Design review of the part built by this model. Coordinates are the model's own, in mm. A direction names the side the tool comes from. Coordinates: 2 decimals unless noted, no trailing zeros. Order: outer loops, then holes, each group sorted by start corner. A loop starts at its lowest first (then second) coordinate and runs counter-clockwise, first axis right, second up. Notation, with made-up numbers: M 89,69 L 135,69 A18 ccw 135,94 Z; hole C -25,7.5 d10. An arc over 180 degrees is marked long. Answer in a Markdown table with one row per item.
from build123d import *

# Parameters (mm, degrees)
SKETCH1_W            = 90.57
SKETCH1_H            = 65.6
BOSS_EXTRUDE1_DEPTH  = 1
SKETCH2_R            = 1.3
CUT_EXTRUDE1_DEPTH   = 112.835973193
SKETCH3_W            = 10.14
SKETCH3_H            = 10.14
SKETCH3_W_2          = 30.4
BOSS_EXTRUDE2_DEPTH  = 8
SKETCH4_W            = 14.4
SKETCH4_H            = 10.82
BOSS_EXTRUDE3_DEPTH  = 6
SKETCH5_W            = 9
SKETCH5_H            = 12
BOSS_EXTRUDE4_DEPTH  = 11
FILLET2_R            = 4.5
SKETCH7_W            = 9
SKETCH7_H            = 3
BOSS_EXTRUDE5_DEPTH  = 11
SKETCH8_R            = 4
BOSS_EXTRUDE6_DEPTH  = 9
SKETCH9_W            = 22.948138565
SKETCH9_H            = 3.071798075
SKETCH9_W_2          = 9.215394227
SKETCH9_H_2          = 3.975268097
SKETCH9_W_3          = 5.149779126
SKETCH9_H_3          = 20.147381496
SKETCH9_W_4          = 3.975268098
SKETCH9_H_4          = 8.94435322
SKETCH9_H_5          = 11.519242784
BOSS_EXTRUDE7_DEPTH  = 5
SKETCH10_W           = 17.979053442
SKETCH10_H           = 12.196845301
BOSS_EXTRUDE8_DEPTH  = 1
SKETCH12_W           = 26.83305966
SKETCH12_H           = 5.142650184
BOSS_EXTRUDE9_DEPTH  = 2.5
SKETCH13_W           = 30.989021763
SKETCH13_H           = 4.427003109
BOSS_EXTRUDE10_DEPTH = 5


with BuildPart() as part:
    # Sketch1 → Boss-Extrude1 (new body)
    with BuildSketch(Plane(origin=(0, 0, 0), x_dir=(1, 0, 0), z_dir=(0, 1, 0))):
        with Locations((45.285, 32.8)):
            Rectangle(SKETCH1_W, SKETCH1_H)
    extrude(amount=BOSS_EXTRUDE1_DEPTH)

    # Sketch2 → Cut-Extrude1 (cut, through all)
    with BuildSketch(Plane(origin=(0, 1, 0), x_dir=(1, 0, 0), z_dir=(0, 1, 0))):
        with Locations(Location((2.36, 2.31, 0), (0, 0, 270))):
            Circle(SKETCH2_R)
        with Locations(Location((3.099, 62.1, 0), (0, 0, 270))):
            Circle(SKETCH2_R)
        with Locations(Location((88.7, 61.87, 0), (0, 0, 270))):
            Circle(SKETCH2_R)
        with Locations(Location((79.55, 1.49, 0), (0, 0, 270))):
            Circle(SKETCH2_R)
    extrude(amount=-CUT_EXTRUDE1_DEPTH, mode=Mode.SUBTRACT)

    # Sketch3 → Boss-Extrude2 (add)
    with BuildSketch(Plane(origin=(0, 1, 0), x_dir=(1, 0, 0), z_dir=(0, 1, 0))):
        with Locations((10.91, 62.53)):
            Rectangle(SKETCH3_W, SKETCH3_H)
        with Locations((33.46, 62.53)):
            Rectangle(SKETCH3_W_2, SKETCH3_H)
    extrude(amount=BOSS_EXTRUDE2_DEPTH)

    # Sketch4 → Boss-Extrude3 (add)
    with BuildSketch(Plane(origin=(0, 1, 0), x_dir=(1, 0, 0), z_dir=(0, 1, 0))):
        with Locations((59.95, 60.19)):
            Rectangle(SKETCH4_W, SKETCH4_H)
    extrude(amount=BOSS_EXTRUDE3_DEPTH)

    # Sketch5 → Boss-Extrude4 (add)
    with BuildSketch(Plane(origin=(0, 1, 0), x_dir=(1, 0, 0), z_dir=(0, 1, 0))):
        with Locations((81.97, 59.6)):
            Rectangle(SKETCH5_W, SKETCH5_H)
    extrude(amount=BOSS_EXTRUDE4_DEPTH)

    # Fillet2
    fillet2_edges = [part.edges().sort_by_distance(p)[0] for p in [
        (86.47, 12, -59.6),
        (77.47, 12, -59.6),
    ]]
    fillet(fillet2_edges, radius=FILLET2_R - 0.0001)  # a hair under: the kernel refuses the full size

    # Sketch7 → Boss-Extrude5 (add)
    with BuildSketch(Plane(origin=(0, 1, 0), x_dir=(1, 0, 0), z_dir=(0, 1, 0))):
        with Locations((81.97, 67.1)):
            Rectangle(SKETCH7_W, SKETCH7_H)
    extrude(amount=BOSS_EXTRUDE5_DEPTH)

    # Sketch8 → Boss-Extrude6 (add)
    with BuildSketch(Plane(origin=(0, 0, -67.6), x_dir=(-1, 0, 0), z_dir=(0, 0, -1))):
        with Locations(Location((-10.91, 5, 0), (0, 0, 270))):
            Circle(SKETCH8_R)
    extrude(amount=BOSS_EXTRUDE6_DEPTH)

    # Sketch9 → Boss-Extrude7 (add)
    with BuildSketch(Plane(origin=(0, 1, 0), x_dir=(1, 0, 0), z_dir=(0, 1, 0))):
        with Locations((34.443359734, 53.839684383)):
            Rectangle(SKETCH9_W, SKETCH9_H)
        with Locations((11.404874166, 47.334700223)):
            Rectangle(SKETCH9_W_2, SKETCH9_H_2)
        with Locations((6.661656549, 22.263407105)):
            Rectangle(SKETCH9_W_3, SKETCH9_H_3)
        with Locations((83.953516952, 39.248643523)):
            Rectangle(SKETCH9_W_4, SKETCH9_H_4)
        with Locations((83.953516952, 28.023028497)):
            Rectangle(SKETCH9_W_4, SKETCH9_H_5)
    extrude(amount=BOSS_EXTRUDE7_DEPTH)

    # Sketch10 → Boss-Extrude8 (add)
    with BuildSketch(Plane(origin=(0, 1, 0), x_dir=(1, 0, 0), z_dir=(0, 1, 0))):
        with Locations((39.18657735, 33.647129386)):
            Rectangle(SKETCH10_W, SKETCH10_H)
    extrude(amount=BOSS_EXTRUDE8_DEPTH)

    # Sketch12 → Boss-Extrude9 (add)
    with BuildSketch(Plane(origin=(0, 1, 0), x_dir=(1, 0, 0), z_dir=(0, 1, 0))):
        with Locations((32.862287194, 2.571325092)):
            Rectangle(SKETCH12_W, SKETCH12_H)
    extrude(amount=BOSS_EXTRUDE9_DEPTH)

    # Sketch13 → Boss-Extrude10 (add)
    with BuildSketch(Plane(origin=(0, 1, 0), x_dir=(1, 0, 0), z_dir=(0, 1, 0))):
        with Locations((39.186577349, 19.462650037)):
            Rectangle(SKETCH13_W, SKETCH13_H)
    extrude(amount=BOSS_EXTRUDE10_DEPTH)


solid = part.part
(1) Add section C-C, the plane x = 59. Give the boundary of the cut face in (y, z).
Return value:
| item | result |
|---|---|
| outline | M 0,-65.6 L 7,-65.6 L 7,-54.78 L 1,-54.78 L 1,0 L 0,0 Z |
(2) For line 1 along X through (y, z) = (0.4, -62.1); line 2 along X through (y, z) = (0.7, -2.31); line 3 along Z through (x, y) = (79.55, 0.5), list the stretches that pass through material, from the lowest coordinate up. Write a range as from..to.
Return value:
| item | result |
|---|---|
| line 1 | x = 0..1.8, 4.4..87.42, 89.98..90.57 |
| line 2 | x = 0..1.06, 3.66..78.54, 80.56..90.57 |
| line 3 | z = -65.6..-2.79, -0.19..0 |
(3) Draft analysis for pull direction Z (two halves, no side actions). For faces 1 (the flat face through (84, 3, -22.263)), 2 (the flat face through (45, 1, -26)), 3 (the cylindrical face through (85.187, 10.647, -59.684)), state which applies: pulls with the +Z half, pulls with the -Z half, needs draft (parallel to the pull), parting line crosses it, or undercut.
Return value:
| item | result |
|---|---|
| face 1 | pulls with the +Z half |
| face 2 | undercut |
| face 3 | needs draft |
(4) For faces 4 (the flat face through (86.47, 5, -63)), 5 (the flat face through (45.917, 3, -54)), 6 (the cylindrical face through (78.753, 10.647, -59.684)), 7 (the flat face through (67.15, 4, -60)), 8 (the flat face through (11, 6, -47)), list the 3-axis set-ups (+Z, -Z, +X, -X, +Y, -Y) from which the entire face can be reached by the end or side of a thin tool; tool diameter is ignored.
Return value:
| item | result |
|---|---|
| face 4 | +Z, -Z, +X, +Y |
| face 5 | +Y |
| face 6 | +Z, +Y |
| face 7 | +Z, -Z, +Y |
| face 8 | +Z, +X, -X, +Y |
(5) Add section A-A, the plane x = 79.55. Give the boundary of the cut face in (y, z), and give its area (3 significant figures).
Return value:
| item | result |
|---|---|
| outline | M 0,-65.6 L 1,-65.6 L 1,-68.6 L 12,-68.6 L 12,-65.6 L 11.29,-65.6 L 11.29,-53.6 L 1,-53.6 L 1,-2.79 L 0,-2.79 Z; M 0,-0.19 L 1,-0.19 L 1,0 L 0,0 Z |
| area | 220 mm2 |
(6) Add section D-D, the plane y = 5. Give the number of separate pieces and of enclosed holes in the cut face, and give its area (3 significant figures).
Return value:
| item | result |
|---|---|
| separate pieces | 10 |
| enclosed holes | 0 |
| area | 1,200 mm2 |
(7) Insertion check: pin 1 Ø5.5 at (x, y) = (64, 3) entering from -Z; pin 2 Ø3 at (y, z) = (6.5, -25.5) entering from -X; pin 3 Ø0.8 at (y, z) = (1.5, -3) entering from -X. Each pin has a flat end and moves straight along its axis. Give the tip position at first contact, or say it passes through.
Return value:
| item | result |
|---|---|
| pin 1 | stops at z = -65.6 |
| pin 2 | stops at x = 4.09 |
| pin 3 | stops at x = 19.45 |
